Build history of the part. All positions in model axes, mm. A direction names the side the tool comes from. Round coordinates to 2 decimals unless told otherwise and drop trailing zeros. Loops run counter-clockwise (first coordinate to the right, second up) from the corner with the lowest first, then second, coordinate; pieces in that order, holes last. Notation, with made-up numbers: M 76.5,42.25 L 114.5,42.25 A4 cw 114.5,48.25 Z; hole C 24,12 d3. An arc over 180 degrees is marked long. One line per item, written item: value.
```python
from build123d import *

# Parameters (mm, degrees)
SKETCH_1_R      = 0.85
SKETCH_1_R_2    = 0.5
SKETCH_1_R_3    = 0.75
EXTRUDE_1_DEPTH = 1.5
FILLET_1_R      = 0.5


with BuildPart() as part:
    # Эскиз1 → Бобышка-Вытянуть1 (new body)
    with BuildSketch(Plane.XY):
        with BuildLine():
            Line((-13, 9.091910703), (-13, 66.908089297))
            ThreePointArc((-13, 66.908089297), (-12.819077862, 67.934149727), (-12.298133329, 68.836452126))
            Line((-12.298133329, 68.836452126), (-5.508214043, 76.928362829))
            ThreePointArc((-5.508214043, 76.928362829), (-4.477935499, 77.718923361), (-3.210080714, 78))
            Line((-3.210080714, 78), (3.5, 78))
            ThreePointArc((3.5, 78), (5.621320344, 77.121320344), (6.5, 75))
            Line((6.5, 75), (6.5, 71.332159566))
            ThreePointArc((6.5, 71.332159566), (9.671404616, 68.918807395), (12, 65.684658438))
            Line((12, 65.684658438), (12, 53.315341562))
            ThreePointArc((12, 53.315341562), (7.657483264, 48.381863913), (1.5, 46.083592135))
            Line((1.5, 46.083592135), (1.5, 39.936491673))
            ThreePointArc((1.5, 39.936491673), (-2.630843406, 41.949941341), (-5.929058411, 38.75))
            Line((-5.929058411, 38.75), (-7, 38.75))
            Line((-7, 38.75), (-7, 37.25))
            Line((-7, 37.25), (-5.929058411, 37.25))
            ThreePointArc((-5.929058411, 37.25), (-2.630843406, 34.050058659), (1.5, 36.063508327))
            Line((1.5, 36.063508327), (1.5, 29.916407865))
            ThreePointArc((1.5, 29.916407865), (7.657483264, 27.618136087), (12, 22.684658438))
            Line((12, 22.684658438), (12, 10.315341562))
            ThreePointArc((12, 10.315341562), (9.671404616, 7.081192605), (6.5, 4.667840434))
            Line((6.5, 4.667840434), (6.5, 1))
            ThreePointArc((6.5, 1), (5.621320344, -1.121320344), (3.5, -2))
            Line((3.5, -2), (-3.210080714, -2))
            ThreePointArc((-3.210080714, -2), (-4.477935499, -1.718923361), (-5.508214043, -0.928362829))
            Line((-5.508214043, -0.928362829), (-12.298133329, 7.163547874))
            ThreePointArc((-12.298133329, 7.163547874), (-12.819077862, 8.065850273), (-13, 9.091910703))
        make_face()
        Circle(SKETCH_1_R, mode=Mode.SUBTRACT)
        with Locations((0, 76)):
            Circle(SKETCH_1_R, mode=Mode.SUBTRACT)
        with Locations((0, 16.5)):
            Circle(SKETCH_1_R_2, mode=Mode.SUBTRACT)
        with Locations((0, 59.5)):
            Circle(SKETCH_1_R_2, mode=Mode.SUBTRACT)
        with Locations((-5, 44.5)):
            Circle(SKETCH_1_R_3, mode=Mode.SUBTRACT)
        with Locations((-5, 31.5)):
            Circle(SKETCH_1_R_3, mode=Mode.SUBTRACT)
    extrude(amount=EXTRUDE_1_DEPTH)

    # Скругление1
    fillet_1_edges = [part.edges().sort_by_distance(p)[0] for p in [
        (1.5, 36.063508327, 0.75),
        (1.5, 39.936491673, 0.75),
    ]]
    fillet(fillet_1_edges, radius=FILLET_1_R)


solid = part.part
```
Item 1: Which spindle directions (+Z, -Z, +X, -X, +Y, -Y) get a long thin tool onto all of the face, cutting with end or side? Do faces 1 (the face through (6.5, 73, 1)), 2 (the face through (5.64, -1.1, 0.74)), 3 (the face through (1.5, 44, 1)). Say none if no direction does.
Check values:
face 1: +Z, -Z, +X, +Y
face 2: +Z, -Z, +X, -Y
face 3: +Z, -Z, +X
Item 2: Wall check: line 1 along Y through (x, z) = (0, 0.5); line 2 along X through (y, z) = (59.5, 0.6); line 3 along X through (y, z) = (76, 1). Give the ranges that are in metal, low to high.
Check values:
line 1: y = -2 to -0.85, 0.85 to 16, 17 to 34.54, 41.46 to 59, 60 to 75.15, 76.85 to 78
line 2: x = -13 to -0.5, 0.5 to 12
line 3: x = -6.29 to -0.85, 0.85 to 6.33
Item 3: Slice it at A-A, the plane x = 5. Give the cut face in (y, z), and give its area (3 significant figures).
Check values:
outline: M -1.6,0 L 29.04,0 L 29.04,1.5 L -1.6,1.5 Z; M 46.96,0 L 77.6,0 L 77.6,1.5 L 46.96,1.5 Z
area: 91.9 mm2
Item 4: Slice it at B-B, the plane y = 31.5. Give the cut face in (x, z).
Check values:
outline: M -13,0 L -5.75,0 L -5.75,1.5 L -13,1.5 Z; M -4.25,0 L 1.5,0 L 1.5,1.5 L -4.25,1.5 Z
Item 5: Pull direction Y, two halves, no side cores. Call faces 4 (the face through (-8.856, 3.061, 0.74)), 5 (the face through (9.63, 68.96, 0.74)), 6 (the face through (-5.098, 32.244, 0.74)): pulls with the +Y half, pulls with the -Y half, needs draft (parallel to the pull), parting line crosses it, or undercut.
Check values:
face 4: pulls with the -Y half
face 5: pulls with the +Y half
face 6: undercut
Item 6: Slice it at C-C, the plane z = 1.1. Give the number of separate pieces and of enclosed holes in the cut face, and give its area (3 significant figures).
Check values:
separate pieces: 1
enclosed holes: 6
area: 1,530 mm2
Item 7: Drop a flat-ended pin along its axis: P1, Ø1.5, axis at x = 0, y = 76, coming from the -Z side. Give the stop position or say it passes through.
Check values:
P1: passes through
